```python
from build123d import *

# Parameters (mm, degrees)
SKETCH2_W                    = 300
SKETCH2_H                    = 150
BOSS_EXTRUDE1_DEPTH          = 10
FILLET1_R                    = 10
M16_TAPPED_HOLE1_D           = 14
M16_TAPPED_HOLE1_CSINK_D     = 16.05
M16_TAPPED_HOLE1_CSINK_ANGLE = 90


with BuildPart() as part:
    # Sketch2 → Boss-Extrude1 (new, symmetric)
    with BuildSketch(Plane(origin=(0, 0, 0), x_dir=(1, 0, 0), z_dir=(0, 1, 0))):
        Rectangle(SKETCH2_W, SKETCH2_H)
    extrude(amount=BOSS_EXTRUDE1_DEPTH, both=True)

    # Fillet1
    fillet1_edges = [part.edges().sort_by_distance(p)[0] for p in [
        (150, 0, 75),
        (-150, 0, 75),
        (-150, 0, -75),
        (150, 0, -75),
    ]]
    fillet(fillet1_edges, radius=FILLET1_R)

    # M16 Tapped Hole1 (through all)
    with Locations(Plane(origin=(-120, 10, -55), x_dir=(0, 0, 1), z_dir=(0, 1, 0))):
        with Locations((0, 0), (0, 240), (110, 240), (110, 0)):
            CounterSinkHole(M16_TAPPED_HOLE1_D / 2, M16_TAPPED_HOLE1_CSINK_D / 2, counter_sink_angle=M16_TAPPED_HOLE1_CSINK_ANGLE)


solid = part.part
```
Here's how the part is built. I have some questions about the finished solid (model axes, mm). Coordinates: 2 decimals unless noted, no trailing zeros. Order: outer loops, then holes, each group sorted by start corner. A loop starts at its lowest first (then second) coordinate and runs counter-clockwise, first axis right, second up.
1) I need wall thicknesses on line 1 (X direction, y = 4, z = -55); line 2 (Z direction, x = -120, y = -0.25). Which ranges of each line are inside material? Lowest first, please.
2) Imagine slicing it at A-A on z = 55. List the corners of the cut face in (x, y) for me (3 decimals), and give its area (3 significant figures).
3) Imagine slicing it at B-B on x = 120. List the corners of the cut face in (y, z) for me (3 decimals).
4) Imagine slicing it at C-C on y = 5.75. List the corners of the cut face in (x, z) for me.
5) Will this pin go through, and if not, where does the flat tip stop? pin 1 (12.5 mm diameter, centred on x = -120, z = -55, fed in from +Y).
6) We'd pull the mould along Z, two halves only. Please class faces 1 (the face through (-126.21, -0.65, 51.77)), 2 (the face through (150, 0, 1)), 3 (the face through (147.15, -0.14, -71.99)): +Z half, -Z half, draft (parallel to the pull), parting line (faces both ways), or undercut.
Response values:
1. line 1: x = -150 to -127, -113 to 113, 127 to 150
1. line 2: z = -75 to -62, -48 to 48, 62 to 75
2. outline: (-150, -10) - (-127, -10) - (-127, 8.975) - (-128.025, 10) - (-150, 10) - close; (-113, -10) - (113, -10) - (113, 8.975) - (111.975, 10) - (-111.975, 10) - (-113, 8.975) - close; (127, -10) - (150, -10) - (150, 10) - (128.025, 10) - (127, 8.975) - close
2. area: 5,440 mm2
3. outline: (-10, -75) - (10, -75) - (10, -63.025) - (8.975, -62) - (-10, -62) - close; (-10, -48) - (8.975, -48) - (10, -46.975) - (10, 46.975) - (8.975, 48) - (-10, 48) - close; (-10, 62) - (8.975, 62) - (10, 63.025) - (10, 75) - (-10, 75) - close
4. outline: (-150, -65) arc R10 ccw to (-140, -75) - (140, -75) arc R10 ccw to (150, -65) - (150, 65) arc R10 ccw to (140, 75) - (-140, 75) arc R10 ccw to (-150, 65) - close; hole circle Ø14 at (-120, -55); hole circle Ø14 at (-120, 55); hole circle Ø14 at (120, -55); hole circle Ø14 at (120, 55)
5. pin 1: passes through
6. face 1: undercut
6. face 2: draft
6. face 3: -Z half
